Design review of the part built by this model. Coordinates are the model's own, in mm. A direction names the side the tool comes from. Give positions to 0.01 mm unless a question says otherwise; leave off trailing zeros. Loops run counter-clockwise (first coordinate to the right, second up) from the corner with the lowest first, then second, coordinate; pieces in that order, holes last. Notation, with made-up numbers: (-23, 87) -> (19, 87) arc R11 cw to (19, 107) -> close; hole circle Ø11 at (67.5, 62.25). An arc over 180 degrees is marked (long way). Answer as CSV lines item,"result".
from build123d import *


with BuildPart() as f1:
    # F0 (on Right) → F1 (revolve)
    with BuildSketch(Plane.YZ):
        with BuildLine():
            Line((-9.532932, 10.287), (-9.532932, 0))
            Line((-9.532932, 0), (-7.373932, 0))
            Line((-7.373932, 0), (6.596068, 0))
            Line((6.596068, 0), (6.596068, 8.4455))
            Line((6.596068, 8.4455), (3.657317, 8.4455))
            Line((3.657317, 8.4455), (0.881068, 8.4455))
            ThreePointArc((0.881068, 8.4455), (0.246068, 7.8105), (-0.388932, 8.4455))
            Line((-0.388932, 8.4455), (-3.165181, 8.4455))
            Line((-3.165181, 8.4455), (-7.373932, 8.4455))
            Line((-7.373932, 8.4455), (-7.373932, 10.287))
            Line((-7.373932, 10.287), (-9.532932, 10.287))
        make_face()
    revolve(axis=Axis((0, -0.388932, 0), (0, 1, 0)))


solid = f1.part
Q1. For faces 1 (the cylindrical face through (2.537, 3.699, 8.056)), 2 (the flat face through (0, -9.533, 0)), list the 3-axis set-ups (+Z, -Z, +X, -X, +Y, -Y) from which the entire face can be reached by the end or side of a thin tool; tool diameter is ignored.
Filled sheet:
face 1,"+Y"
face 2,"+Z, -Z, +X, -X, -Y"
Q2. We need section D-D, the plane z = 9. State the section outline as (x, y) points.
Filled sheet:
outline,"(-4.98, -9.53) -> (4.98, -9.53) -> (4.98, -7.37) -> (-4.98, -7.37) -> close"
Q3. We need section C-C, the plane y = -1. State the section outline as (x, z) points, and give its area (3 significant figures).
Filled sheet:
outline,"circle Ø16.89 at (0, 0)"
area,"224 mm^2"
Q4. We need section A-A, the plane z = 0. State the section outline as (x, y) points (1 decimal), and give its area (3 significant figures).
Filled sheet:
outline,"(-10.3, -9.5) -> (10.3, -9.5) -> (10.3, -7.4) -> (8.4, -7.4) -> (8.4, -0.4) arc R0.6 cw to (8.4, 0.9) -> (8.4, 6.6) -> (-8.4, 6.6) -> (-8.4, 0.9) arc R0.6 cw to (-8.4, -0.4) -> (-8.4, -7.4) -> (-10.3, -7.4) -> close"
area,"279 mm^2"
Q5. To check wall thickness, follow probe 1 along X at (y, z) = (-4.25, 0); probe 2 along Y at (x, z) = (3.75, -7.5); probe 3 along Y at (x, z) = (6, -6.75). State the ranges of each line that lie inside material, in increasing order. Write a range as from..to.
Filled sheet:
probe 1,"x = -8.45..8.45"
probe 2,"y = -9.53..-0.39, 0.88..6.6"
probe 3,"y = -9.53..-7.37"
Q6. We need section B-B, the plane x = 0. State the section outline as (y, z) points (1 decimal), and give its area (3 significant figures).
Filled sheet:
outline,"(-9.5, -10.3) -> (-7.4, -10.3) -> (-7.4, -8.4) -> (-0.4, -8.4) arc R0.6 cw to (0.9, -8.4) -> (6.6, -8.4) -> (6.6, 8.4) -> (0.9, 8.4) arc R0.6 cw to (-0.4, 8.4) -> (-7.4, 8.4) -> (-7.4, 10.3) -> (-9.5, 10.3) -> close"
area,"279 mm^2"
Q7. Clearance check with flat-ended pins moving along their axes: pin 1 Ø1 at (y, z) = (0.5, -1) entering from -X; pin 2 Ø6 at (x, y) = (2.5, -6) entering from -Z; pin 3 Ø1 at (y, z) = (-6.5, -4) entering from +X; pin 4 Ø5 at (x, y) = (-5, 4) entering from +Z. State where each tip first meets the part, or that it passes through.
Filled sheet:
pin 1,"stops at x = -8.42"
pin 2,"stops at z = -10.29"
pin 3,"stops at x = 7.69"
pin 4,"stops at z = 8.07"
